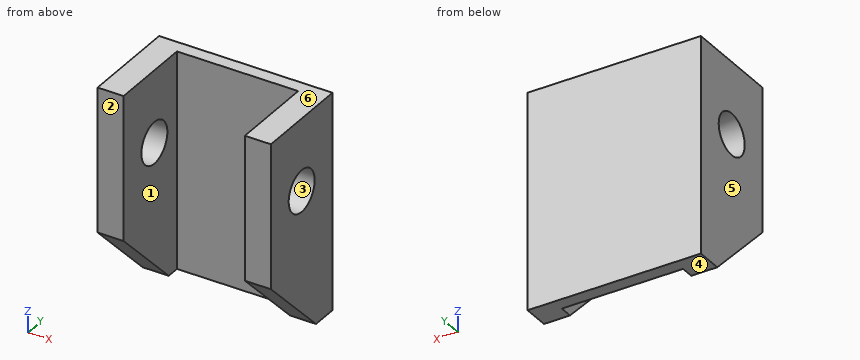
```python
from build123d import *

# Parameters (mm, degrees)
F0_W     = 67.0874267817
F0_H     = 83.7676301599
F1_DEPTH = 38.1
F2_W     = 46.9245351851
F2_H     = 83.7676301599
F3_DEPTH = 33.02
F4_SIZE  = 27.94
F5_SIZE  = 27.94
F6_R     = 8.0338499756
F7_DEPTH = 67.0884267817


with BuildPart() as f1:
    # F0 (on Front) → F1 (new body)
    with BuildSketch(Plane.XZ):
        Rectangle(F0_W, F0_H)
    extrude(amount=F1_DEPTH)

    # F2 (on face) → F3 (cut)
    with BuildSketch(Plane.XZ.offset(38.1)):
        Rectangle(F2_W, F2_H)
    extrude(amount=-F3_DEPTH, mode=Mode.SUBTRACT)

    # F4
    f4_edges = [f1.edges().sort_by_distance(p)[0] for p in [
        (28.50299, -38.1, -41.883815),
    ]]
    chamfer(f4_edges, length=F4_SIZE)

    # F5
    f5_edges = [f1.edges().sort_by_distance(p)[0] for p in [
        (-28.50299, -38.1, -41.883815),
    ]]
    chamfer(f5_edges, length=F5_SIZE)

    # F6 (on face) → F7 (cut, through all)
    with BuildSketch(Plane.YZ.offset(33.5437133908)):
        with Locations((-19.05, 13.97)):
            Circle(F6_R)
    extrude(amount=-F7_DEPTH, mode=Mode.SUBTRACT)


solid = f1.part
```
Could you check a few things on this model? Use its own coordinates, in mm. Face numbers are marked on the shaded views. A direction names the side the tool comes from. Round coordinates to 2 decimals unless told otherwise and drop trailing zeros. Loops run counter-clockwise (first coordinate to the right, second up) from the corner with the lowest first, then second, coordinate; pieces in that order, holes last. Notation, with made-up numbers: M 1,48.25 L 6,48.25 A26 ccw 6,72.25 Z; hole C 29.5,48 d11. An arc over 180 degrees is marked long. Put each result on its own line as item: value.
Q1. I need wall thicknesses on probe 1 along X at (y, z) = (-14.5, -19); probe 2 along Y at (x, z) = (21, 36.5); probe 3 along Y at (x, z) = (-26, 13). Which ranges of each line are inside material? Lowest first, please.
Check result:
probe 1: -33.54 to -23.46, 23.46 to 33.54
probe 2: -5.08 to 0
probe 3: -38.1 to -27.03, -11.07 to 0
Q2. For pin 1 (4 mm diameter, centred on x = -3, z = 4.5, fed in from -Y); pin 2 (10 mm diameter, centred on x = 12, y = -11.5, fed in from -Z), each with a flat end and sliding along its axis, tell me the tip position at first contact or that it passes through.
Check result:
pin 1: y = -5.08
pin 2: through
Q3. On a 3-axis mill with a long thin cutter (end or side, diameter ignored), from which of +Z, -Z, +X, -X, +Y, -Y can I reach the whole of each face in a straight line? I mean the marked faces 1 and 2. Say none if no direction works.
Check result:
face 1: +Z, -Z, -Y
face 2: +Z, -Z, +X, -X, -Y
Q4. Imagine slicing it at C-C (y = -19.05). Write out the boundary of the cut face in (x, z), then the cut area to 3 significant figures.
Check result:
outline: M -33.54,-32.99 L -23.46,-32.99 L -23.46,5.94 L -33.54,5.94 Z; M -33.54,22 L -23.46,22 L -23.46,41.88 L -33.54,41.88 Z; M 23.46,-32.99 L 33.54,-32.99 L 33.54,5.94 L 23.46,5.94 Z; M 23.46,22 L 33.54,22 L 33.54,41.88 L 23.46,41.88 Z
area: 1,190 mm2
Q5. Imagine slicing it at D-D (y = -35). Write out the boundary of the cut face in (x, z).
Check result:
outline: M -33.54,-17.04 L -23.46,-17.04 L -23.46,41.88 L -33.54,41.88 Z; M 23.46,-17.04 L 33.54,-17.04 L 33.54,41.88 L 23.46,41.88 Z
Q6. Imagine slicing it at A-A (x = -27.5). Write out the boundary of the cut face in (y, z), then the cut area to 3 significant figures.
Check result:
outline: M -38.1,-13.94 L -10.16,-41.88 L 0,-41.88 L 0,41.88 L -38.1,41.88 Z; hole C -19.05,13.97 d16.07
area: 2,600 mm2
Q7. Thinking about a two-plate mould opening in Z: for the marked faces 3, 4, 5 and 6, which applies, released by +Z, released by -Z, zero draft, split by the parting line, or undercut?
Check result:
face 3: undercut
face 4: released by -Z
face 5: zero draft
face 6: released by +Z
Q8. Imagine slicing it at B-B (z = 13.97). Write out the boundary of the cut face in (x, y).
Check result:
outline: M -33.54,-38.1 L -23.46,-38.1 L -23.46,-27.08 L -33.54,-27.08 Z; M -33.54,-11.02 L -23.46,-11.02 L -23.46,-5.08 L 23.46,-5.08 L 23.46,-11.02 L 33.54,-11.02 L 33.54,0 L -33.54,0 Z; M 23.46,-38.1 L 33.54,-38.1 L 33.54,-27.08 L 23.46,-27.08 Z
